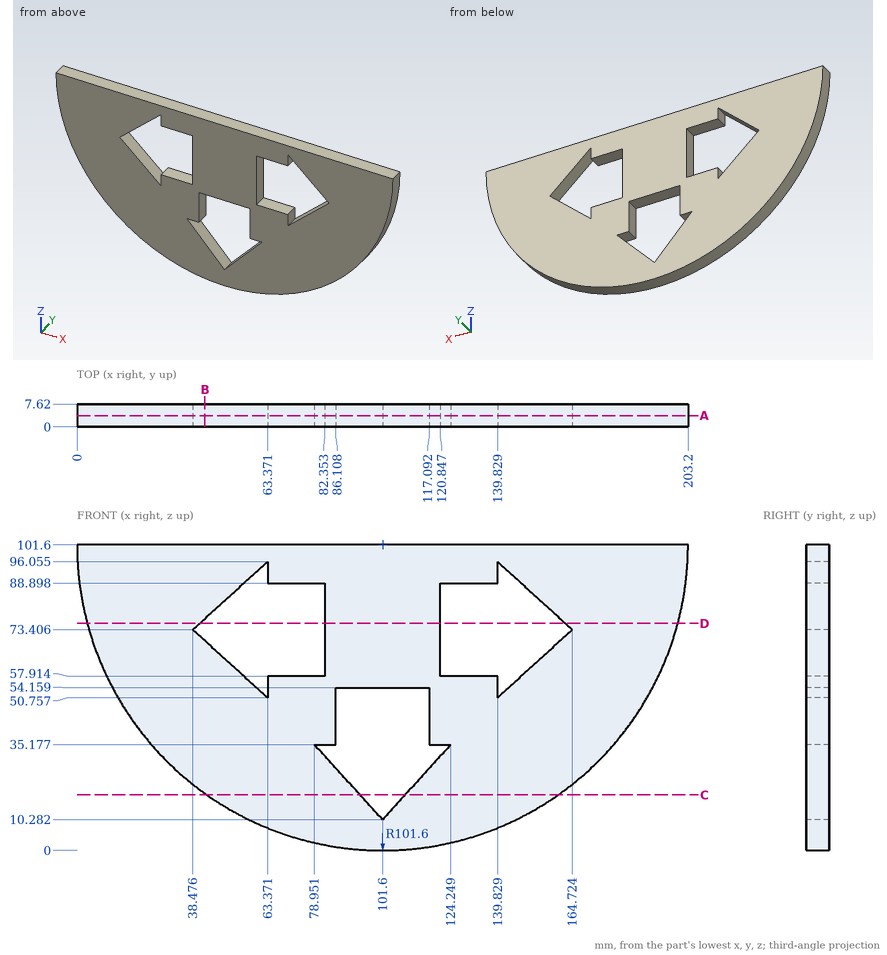
Print and shaded views of the part. All mm, measured from the part's lowest x, y and z. Coordinates: 2 decimals unless noted, no trailing zeros. Loops run counter-clockwise (first coordinate to the right, second up) from the corner with the lowest first, then second, coordinate; pieces in that order, holes last. Notation, with made-up numbers: (18, 44) -> (52, 44) arc R17 ccw to (52, 74) -> close; hole circle Ø2 at (17.25, -27). An arc over 180 degrees is marked (long way). Use a Markdown table: item, result. Add a question column.
Item 1: Band-saw the part on D-D on z = 75.5. Write the cut outline in (x, y), plus the area to 3 significant figures.
Item 2: Band-saw the part on A-A on y = 3.75. Write the cut outline in (x, z) (1 decimal).
Item 3: Band-saw the part on C-C on z = 18.5. Write the cut outline in (x, y) (1 decimal), plus the area to 3 significant figures.
Item 4: Probe probe 1 along X at (y, z) = (2.25, 80.5) (1 decimal); probe 2 along X at (y, z) = (1.5, 91.5) (1 decimal); probe 3 along Z at (x, y) = (124, 7.25) (1 decimal). List the from-to ranges inside material, lowest first.
Item 5: Flat gauge pins, fed straight in: P1, Ø2.5, axis at y = 3, z = 66.5, coming from the +X side (1 decimal); P2, Ø3.5, axis at y = 2.5, z = 53, coming from the -X side; P3, Ø3, axis at y = 2, z = 42.5, coming from the +X side (1 decimal). Where does each tip first touch, or does it go through?
Item 6: Band-saw the part on B-B on x = 42.5. Write the cut outline in (y, z) (1 decimal), plus the area to 3 significant figures.
Geometry says:
| question | item | result |
|---|---|---|
| 1 | outline | (3.41, 0) -> (40.78, 0) -> (40.78, 7.62) -> (3.41, 7.62) -> close; (82.35, 0) -> (120.85, 0) -> (120.85, 7.62) -> (82.35, 7.62) -> close; (162.42, 0) -> (199.79, 0) -> (199.79, 7.62) -> (162.42, 7.62) -> close |
| 1 | area | 863 mm² |
| 2 | outline | (0, 101.6) arc R101.6 ccw to (203.2, 101.6) -> close; hole (38.5, 73.4) -> (63.4, 50.8) -> (63.4, 57.9) -> (82.4, 57.9) -> (82.4, 88.9) -> (63.4, 88.9) -> (63.4, 96.1) -> close; hole (79, 35.2) -> (101.6, 10.3) -> (124.2, 35.2) -> (117.1, 35.2) -> (117.1, 54.2) -> (86.1, 54.2) -> (86.1, 35.2) -> close; hole (120.8, 57.9) -> (139.8, 57.9) -> (139.8, 50.8) -> (164.7, 73.4) -> (139.8, 96.1) -> (139.8, 88.9) -> (120.8, 88.9) -> close |
| 3 | outline | (43.1, 0) -> (94.1, 0) -> (94.1, 7.6) -> (43.1, 7.6) -> close; (109.1, 0) -> (160.1, 0) -> (160.1, 7.6) -> (109.1, 7.6) -> close |
| 3 | area | 777 mm² |
| 4 | probe 1 | 2.2 to 46.3, 82.4 to 120.8, 156.9 to 201 |
| 4 | probe 2 | 0.5 to 58.4, 63.4 to 139.8, 144.8 to 202.7 |
| 4 | probe 3 | 2.5 to 34.9, 35.2 to 57.9, 88.9 to 101.6 |
| 5 | P1 | x = 197.4 |
| 5 | P2 | x = 11.45 |
| 5 | P3 | x = 185.3 |
| 6 | outline | (0, 19) -> (7.6, 19) -> (7.6, 69.7) -> (0, 69.7) -> close; (0, 77.1) -> (7.6, 77.1) -> (7.6, 101.6) -> (0, 101.6) -> close |
| 6 | area | 574 mm² |
